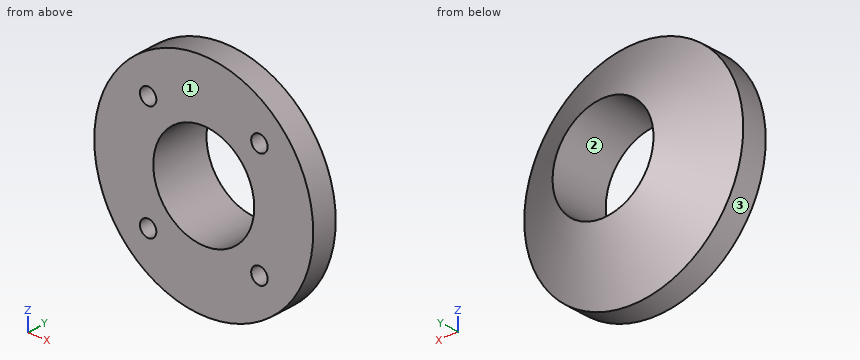
```python
from build123d import *

# Parameters (mm, degrees)
SKETCH001_R  = 1.25
POCKET_DEPTH = 3


with BuildPart() as part:
    # Sketch → Revolution (revolve)
    with BuildSketch(Plane.XY):
        Polygon((7.7, 0), (16.7, 0), (16.7, 3.803848), (7.7, 9), align=None)
    revolve(axis=Axis((0, 0, 0), (0, 1, 0)))

    # Sketch001 (on Face1 of Revolution) → Pocket (cut)
    with BuildSketch(Plane.XZ):
        with Locations((-8.485281, 8.485281)):
            Circle(SKETCH001_R)
        with Locations((8.485281, 8.485281)):
            Circle(SKETCH001_R)
        with Locations((8.485281, -8.485281)):
            Circle(SKETCH001_R)
        with Locations((-8.485281, -8.485281)):
            Circle(SKETCH001_R)
    extrude(amount=-POCKET_DEPTH, mode=Mode.SUBTRACT)


solid = part.part
```
Input: part model. Units: mm. Frame: model coordinates. Face numbers are marked on the shaded views. Coordinates: 2 decimals unless noted, no trailing zeros. Loops run counter-clockwise (first coordinate to the right, second up) from the corner with the lowest first, then second, coordinate; pieces in that order, holes last. Notation, with made-up numbers: M -13,17 L 29,17 A15 cw 29,30 Z; hole C 9.5,-38 d7. An arc over 180 degrees is marked long. One line per item, written item: value.
(1) Section C-C (y = 2). Output: boundary loops of the cut face in (x, z), and give its area (3 significant figures).
Filled in:
outline: C 0,0 d33.4; hole C -8.49,-8.49 d2.5; hole C -8.49,8.49 d2.5; hole C 0,0 d15.4; hole C 8.49,-8.49 d2.5; hole C 8.49,8.49 d2.5
area: 670 mm^2
(2) Section B-B (z = 0). Output: boundary loops of the cut face in (x, y), and give its area (3 significant figures).
Filled in:
outline: M -16.7,0 L -7.7,0 L -7.7,9 L -16.7,3.8 Z; M 7.7,0 L 16.7,0 L 16.7,3.8 L 7.7,9 Z
area: 115 mm^2
(3) Section A-A (x = 0). Output: boundary loops of the cut face in (y, z), and give its area (3 significant figures).
Filled in:
outline: M 0,-16.7 L 3.8,-16.7 L 9,-7.7 L 0,-7.7 Z; M 0,7.7 L 9,7.7 L 3.8,16.7 L 0,16.7 Z
area: 115 mm^2
(4) Pull-direction query (Z, two-part tool) for the marked faces 1, 2 and 3; classes: +Z half, -Z half, draft (parallel to the pull), parting line (faces both ways), or undercut.
Filled in:
face 1: draft
face 2: undercut
face 3: parting line
(5) Line query: line 1 along Z through (x, y) = (0, 3.5); line 2 along X through (y, z) = (4.75, 0); line 3 along X through (y, z) = (6.75, 0). Output: solid intervals per line, ascending. Write a range as from..to.
Filled in:
line 1: -16.7..-7.7, 7.7..16.7
line 2: -15.06..-7.7, 7.7..15.06
line 3: -11.6..-7.7, 7.7..11.6
(6) Section D-D (y = 4.5). Output: boundary loops of the cut face in (x, z), and give its area (3 significant figures).
Filled in:
outline: C 0,0 d30.99; hole C 0,0 d15.4
area: 568 mm^2
(7) Pin query (flat end, axial travel): pin 1 (1.5 mm diameter, centred on x = 8.49, z = 8.49, fed in from +Y); pin 2 (1.5 mm diameter, centred on x = 10, y = 5.5, fed in from +Z); pin 3 (5 mm diameter, centred on x = 7.5, y = 3.5, fed in from -Z); pin 4 (4 mm diameter, centred on x = -2.5, z = 3, fed in from -Y). Return the tip coordinate at first contact, or that it passes through.
Filled in:
pin 1: y = 6.95
pin 2: z = 11.38
pin 3: z = -15.93
pin 4: through
